Read the model definition and answer for the solid it produces. Units are mm, in the model's axes. A direction names the side the tool comes from. Round coordinates to 2 decimals unless told otherwise and drop trailing zeros. Order: outer loops, then holes, each group sorted by start corner. A loop starts at its lowest first (then second) coordinate and runs counter-clockwise, first axis right, second up. Notation, with made-up numbers: (9, 74.5) -> (67, 74.5) arc R13 cw to (67, 79.5) -> close; hole circle Ø11 at (54, 4.5). An arc over 180 degrees is marked (long way). Use a Markdown table: item, result. Add a question column.
1. Consider L1, parallel to X at y = 10, z = 0.2; L2, parallel to Y at x = 33, z = 2.05; L3, parallel to Y at x = 19, z = 0.5 (3 decimals). Determine where each line is inside the solid, lowest interval first. Write a range as [from, to].
2. The mould has two halves that part along Y. Classify faces 3 (the face through (3.81, 86, 2)), 4 (the face through (-4.343, 43, 2)), 5 (the face through (0, 14, 2)), 6 (the face through (47, -4.343, 2)): +Y half, -Y half, draft (parallel to the pull), parting line (faces both ways), or undercut.
3. Given pin 1 (1.6 mm diameter, centred on x = 29.5, z = 2.5, fed in from -Y), flat-ended and moving along its own axis, determine where the tip first touches the part or whether it passes through.
4. For faces 1 (the face through (16.662, 12, 2)), 2 (the face through (28, 64, 0)), determine the directions among +Z, -Z, +X, -X, +Y, -Y from which every point of the face is accessible in a straight line to the end or side of a thin tool.
5. Section C-C, the plane x = 13.5 is taken. Give the vertices of the cut face in (y, z) (3 decimals), then the cut area to 3 significant figures.
6. Section A-A, the plane x = 34.5 is taken. Give the vertices of the cut face in (y, z) (3 decimals).
7. Section D-D, the plane x = 1 is taken. Give the vertices of the cut face in (y, z) (3 decimals), then the cut area to 3 significant figures.
8. Section B-B, the plane y = 43 is taken. Give the vertices of the cut face in (x, z) (3 decimals).
```python
from build123d import *

# Parameters (mm, degrees)
SKETCH1_R           = 1.397
SKETCH1_W           = 12.7
SKETCH1_H           = 1.8034
SKETCH1_W_2         = 3.175
SKETCH1_H_2         = 4.953
SKETCH1_W_3         = 56.134
SKETCH1_H_3         = 16.7894
SKETCH1_W_4         = 48.514
BOSS_EXTRUDE1_DEPTH = 3.175


with BuildPart() as part:
    # Sketch1 → Boss-Extrude1 (new body)
    with BuildSketch(Plane.XY):
        with BuildLine():
            Line((36.9824, 15.1384), (36.9824, -4.3434))
            Line((36.9824, -4.3434), (57.9374, -4.3434))
            ThreePointArc((57.9374, -4.3434), (59.733451224, -3.599451224), (60.4774, -1.8034))
            Line((60.4774, -1.8034), (60.4774, 86.7664))
            ThreePointArc((60.4774, 86.7664), (59.733451224, 88.562451224), (57.9374, 89.3064))
            Line((57.9374, 89.3064), (-1.8034, 89.3064))
            ThreePointArc((-1.8034, 89.3064), (-3.599451224, 88.562451224), (-4.3434, 86.7664))
            Line((-4.3434, 86.7664), (-4.3434, -1.8034))
            ThreePointArc((-4.3434, -1.8034), (-3.599451224, -3.599451224), (-1.8034, -4.3434))
            Line((-1.8034, -4.3434), (21.717, -4.3434))
            Line((21.717, -4.3434), (21.717, 8.255))
            Line((21.717, 8.255), (16.6624, 8.255))
            Line((16.6624, 8.255), (16.6624, 15.1384))
            Line((16.6624, 15.1384), (36.9824, 15.1384))
        make_face()
        with Locations((3.556, 3.556)):
            Circle(SKETCH1_R, mode=Mode.SUBTRACT)
        with Locations((9.652, -0.9017)):
            Rectangle(SKETCH1_W, SKETCH1_H, mode=Mode.SUBTRACT)
        with Locations((8.0137, 10.8077)):
            Rectangle(SKETCH1_W_2, SKETCH1_H_2, mode=Mode.SUBTRACT)
        with Locations((46.482, -0.9017)):
            Rectangle(SKETCH1_W, SKETCH1_H, mode=Mode.SUBTRACT)
        with Locations((52.578, 3.556)):
            Circle(SKETCH1_R, mode=Mode.SUBTRACT)
        Polygon((49.784, 20.4724), (0, 20.4724), (0, 6.35), (-1.8034, 6.35), (-1.8034, 46.863), (0, 46.863), (0, 58.42), (23.876, 58.42), (23.876, 63.246), (40.259, 63.246), (40.259, 58.42), (56.134, 58.42), (56.134, 46.863), (57.9374, 46.863), (57.9374, 6.35), (56.134, 6.35), (56.134, 6.731), (49.784, 6.731), align=None, mode=Mode.SUBTRACT)
        with Locations((28.067, 74.8157)):
            Rectangle(SKETCH1_W_3, SKETCH1_H_3, mode=Mode.SUBTRACT)
        with Locations((28.067, 85.8647)):
            Rectangle(SKETCH1_W_4, SKETCH1_H, mode=Mode.SUBTRACT)
        with Locations((3.556, 61.595)):
            Circle(SKETCH1_R, mode=Mode.SUBTRACT)
        with Locations((52.578, 61.595)):
            Circle(SKETCH1_R, mode=Mode.SUBTRACT)
    extrude(amount=BOSS_EXTRUDE1_DEPTH)


solid = part.part
```
Verdict:
| question | item | result |
|---|---|---|
| 1 | L1 | x = [-4.34, -1.8], [0, 6.43], [9.6, 16.66], [36.98, 49.78], [57.94, 60.48] |
| 1 | L2 | y = [15.14, 20.47], [63.25, 66.42], [83.21, 84.96], [86.77, 89.31] |
| 1 | L3 | y = [-4.343, 8.255], [15.138, 20.472], [58.42, 66.421], [83.21, 84.963], [86.766, 89.306] |
| 2 | face 3 | undercut |
| 2 | face 4 | draft |
| 2 | face 5 | undercut |
| 2 | face 6 | -Y half |
| 3 | pin 1 | stops at y = 15.14 |
| 4 | face 1 | +Z, -Z |
| 4 | face 2 | -Z, +X, -X, +Y, -Y |
| 5 | outline | (-4.343, 0) -> (-1.803, 0) -> (-1.803, 3.175) -> (-4.343, 3.175) -> close; (0, 0) -> (20.472, 0) -> (20.472, 3.175) -> (0, 3.175) -> close; (58.42, 0) -> (66.421, 0) -> (66.421, 3.175) -> (58.42, 3.175) -> close; (83.21, 0) -> (84.963, 0) -> (84.963, 3.175) -> (83.21, 3.175) -> close; (86.766, 0) -> (89.306, 0) -> (89.306, 3.175) -> (86.766, 3.175) -> close |
| 5 | area | 112 mm2 |
| 6 | outline | (15.138, 0) -> (20.472, 0) -> (20.472, 3.175) -> (15.138, 3.175) -> close; (63.246, 0) -> (66.421, 0) -> (66.421, 3.175) -> (63.246, 3.175) -> close; (83.21, 0) -> (84.963, 0) -> (84.963, 3.175) -> (83.21, 3.175) -> close; (86.766, 0) -> (89.306, 0) -> (89.306, 3.175) -> (86.766, 3.175) -> close |
| 7 | outline | (-4.343, 0) -> (20.472, 0) -> (20.472, 3.175) -> (-4.343, 3.175) -> close; (58.42, 0) -> (66.421, 0) -> (66.421, 3.175) -> (58.42, 3.175) -> close; (83.21, 0) -> (89.306, 0) -> (89.306, 3.175) -> (83.21, 3.175) -> close |
| 7 | area | 124 mm2 |
| 8 | outline | (-4.343, 0) -> (-1.803, 0) -> (-1.803, 3.175) -> (-4.343, 3.175) -> close; (57.937, 0) -> (60.477, 0) -> (60.477, 3.175) -> (57.937, 3.175) -> close |
